The model under review builds one solid part; all positions refer to its coordinate system, in mm. Face numbers are marked on the shaded views. A direction names the side the tool comes from. Give positions to 0.01 mm unless a question says otherwise; leave off trailing zeros. Order: outer loops, then holes, each group sorted by start corner. A loop starts at its lowest first (then second) coordinate and runs counter-clockwise, first axis right, second up.
Autodesk Inventor part; units mm, degrees
ref_plane "YZ Plane" through (0, 0, 0) normal (1, 0, 0) x (0, 1, 0)
ref_plane "XZ Plane" through (0, 0, 0) normal (0, 1, 0) x (-1, 0, 0)
ref_plane "XY Plane" through (0, 0, 0) normal (0, 0, 1) x (1, 0, 0)
sketch "スケッチ1" plane through (0, 0, 0) normal (0, 0, 1) x (1, 0, 0)
  circle A0 centre (0, 0) radius 1.5
  dimension "d0" = 3
extrude "押し出し1" add sketch "スケッチ1" along normal blind 16
thread "ねじ1"
sketch "スケッチ2" plane through (0, 0, 16) normal (0, 0, 1) x (1, 0, 0)
  circle A0 centre (0, 0) radius 3
  dimension "d5" = 6
extrude "押し出し2" add sketch "スケッチ2" against normal blind 1.75
chamfer "面取り1" distance 1.5 angle 45 1 edges at (-3, 0, 14.25)
sketch "スケッチ3" plane through (0, 0, 16) normal (0, 0, 1) x (1, 0, 0)
  line L0 (0, 1.1547) -> (1, 0.5774)
  line L1 (1, 0.5774) -> (1, -0.5774)
  line L2 (1, -0.5774) -> (0, -1.1547)
  line L3 (0, -1.1547) -> (-1, -0.5774)
  line L4 (-1, -0.5774) -> (-1, 0.5774)
  line L5 (-1, 0.5774) -> (0, 1.1547)
  point P0 (0, 0)
  point P1 (0, 0)
  dimension "d11" = 2
extrude "押し出し3" cut sketch "スケッチ3" against normal blind 1.5
properties part number "m3皿ネジ16" material "鉄 灰色"
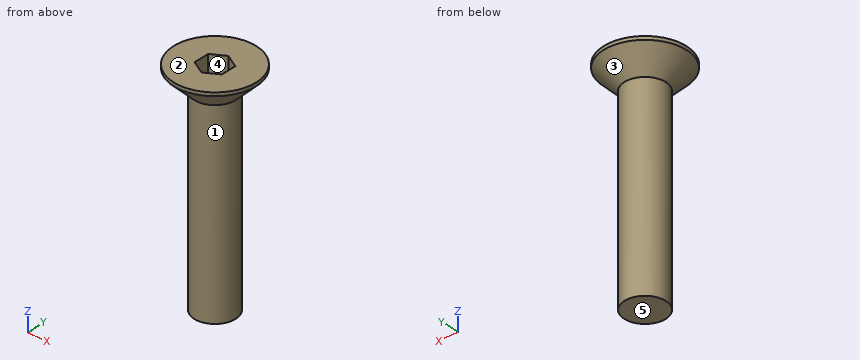
Item 1: Take a section at B-B (z = 10). Give the boundary of the cut face in (x, y).
Values found:
outline: circle Ø3 at (0, 0)
Item 2: Clearance check with flat-ended pins moving along their axes: pin 1 Ø0.9 at (y, z) = (0, 15) entering from -X; pin 2 Ø3 at (x, z) = (1, 12.5) entering from +Y; pin 3 Ø0.9 at (y, z) = (0, 15) entering from +X. State where each tip first meets the part, or that it passes through.
Values found:
pin 1: stops at x = -2.7
pin 2: stops at y = 1.5
pin 3: stops at x = 2.7
Item 3: For line 1 (X direction, y = 0, z = 6.25); line 2 (Z direction, x = 0.75, y = -0.4); line 3 (Y direction, x = -0.2, z = 12), list the stretches that pass through material, from the lowest coordinate up.
Values found:
line 1: x = -1.5 to 1.5
line 2: z = 0 to 14.5
line 3: y = -1.49 to 1.49
Item 4: For the marked faces 1 and 2, list the 3-axis set-ups (+Z, -Z, +X, -X, +Y, -Y) from which the entire face can be reached by the end or side of a thin tool; tool diameter is ignored.
Values found:
face 1: -Z
face 2: +Z, +X, -X, +Y, -Y
Item 5: Draft analysis for pull direction X (two halves, no side actions). For the marked faces 3, 4 and 5, state which applies: released by +X, released by -X, zero draft, split by the parting line, or undercut.
Values found:
face 3: split by the parting line
face 4: undercut
face 5: zero draft
